The model under review builds one solid part; all positions refer to its coordinate system, in mm. A direction names the side the tool comes from. Give positions to 0.01 mm unless a question says otherwise; leave off trailing zeros. Order: outer loops, then holes, each group sorted by start corner. A loop starts at its lowest first (then second) coordinate and runs counter-clockwise, first axis right, second up.
```python
from build123d import *

# Parameters (mm, degrees)
F0_R     = 6.35
F1_DEPTH = 19.05


with BuildPart() as f1:
    # F0 (on Right) → F1 (new body)
    with BuildSketch(Plane.YZ):
        with BuildLine():
            Line((334.807445, -196.726841), (333.773435, -165.933012))
            ThreePointArc((333.773435, -165.933012), (128.220826, 292.742264), (-339.662255, 476.373159))
            Line((-339.662255, 476.373159), (-377.762255, 476.373159))
            Line((-377.762255, 476.373159), (-377.762255, -196.726841))
            Line((-377.762255, -196.726841), (314.387745, -196.726841))
            Line((314.387745, -196.726841), (334.807445, -196.726841))
        make_face()
        with BuildLine():
            ThreePointArc((-339.326565, 438.274146), (101.046912, 266.007515), (295.615862, -164.976841))
            Line((295.615862, -164.976841), (-339.326565, -164.976841))
            Line((-339.326565, -164.976841), (-339.326565, 438.274146))
        make_face(mode=Mode.SUBTRACT)
        with Locations((295.538976, -30.528007)):
            Circle(F0_R, mode=Mode.SUBTRACT)
        with Locations((234.36105, 124.383493)):
            Circle(F0_R, mode=Mode.SUBTRACT)
        with Locations((-350.040551, 457.090986)):
            Circle(F0_R, mode=Mode.SUBTRACT)
        with Locations((-143.276888, 429.635451)):
            Circle(F0_R, mode=Mode.SUBTRACT)
        with Locations((135.900178, 258.16555)):
            Circle(F0_R, mode=Mode.SUBTRACT)
        with Locations((7.055922, 362.096482)):
            Circle(F0_R, mode=Mode.SUBTRACT)
    extrude(amount=F1_DEPTH)


solid = f1.part
```
Item 1: Take a section at A-A (z = 66). Give the boundary of the cut face in (x, y).
Values found:
outline: (0, -377.76) - (19.05, -377.76) - (19.05, -339.33) - (0, -339.33) - close; (0, 242.15) - (19.05, 242.15) - (19.05, 283.6) - (0, 283.6) - close
Item 2: Draft analysis for pull direction Z (two halves, no side actions). For faces 3 (the flat face through (9, -26, -196.727)), 4 (the flat face through (9, -339.327, 132)), 5 (the cylindrical face through (9.39, 133.42, 287.73)), 6 (the flat face through (9, -17, -164.977)), state which applies: released by +Z, released by -Z, zero draft, split by the parting line, or undercut.
Values found:
face 3: released by -Z
face 4: undercut
face 5: released by +Z
face 6: undercut
Item 3: For faces 1 (the flat face through (9, -377.762, 145)), 2 (the cylindrical face through (9.392, 96.1, 270.656)), list the 3-axis set-ups (+Z, -Z, +X, -X, +Y, -Y) from which the entire face can be reached by the end or side of a thin tool; tool diameter is ignored.
Values found:
face 1: +Z, -Z, +X, -X, -Y
face 2: +X, -X
Item 4: Take a section at C-C (x = 14.25). Give the boundary of the cut face in (y, z).
Values found:
outline: (-377.76, -196.73) - (334.81, -196.73) - (333.77, -165.93) arc R664.68 ccw to (-339.66, 476.37) - (-377.76, 476.37) - close; hole circle Ø12.7 at (-350.04, 457.09); hole (-339.33, -164.98) - (295.62, -164.98) arc R626.58 ccw to (-339.33, 438.27) - close; hole circle Ø12.7 at (-143.28, 429.64); hole circle Ø12.7 at (7.06, 362.1); hole circle Ø12.7 at (135.9, 258.17); hole circle Ø12.7 at (234.36, 124.38); hole circle Ø12.7 at (295.54, -30.53)
Item 5: For line 1 (Y direction, x = 8, z = -162); line 2 (Z direction, x = 11.75, y = -337); line 3 (Z direction, x = 13.25, y = -315), list the stretches that pass through material, from the lowest coordinate up.
Values found:
line 1: y = -377.76 to -339.33, 295.5 to 333.63
line 2: z = -196.73 to -164.98, 438.3 to 476.4
line 3: z = -196.73 to -164.98, 438.14 to 476.25
Item 6: Take a section at B-B (y = -272). Give the boundary of the cut face in (x, z), and give its area (3 significant figures).
Values found:
outline: (0, -196.73) - (19.05, -196.73) - (19.05, -164.98) - (0, -164.98) - close; (0, 435.6) - (19.05, 435.6) - (19.05, 473.85) - (0, 473.85) - close
area: 1,330 mm2
Item 7: Clearance check with flat-ended pins moving along their axes: pin 1 Ø9.5 at (x, z) = (11, 87) entering from +Y; pin 2 Ø10 at (x, y) = (10.5, 66.5) entering from +Z; pin 3 Ø1.5 at (x, z) = (16.5, 157) entering from +Y. State where each tip first meets the part, or that it passes through.
Values found:
pin 1: stops at y = 276.62
pin 2: stops at z = 348.52
pin 3: stops at y = 237.91
